from build123d import *

# Parameters (mm, degrees)
F1_DEPTH  = 45
F3_D      = 5
F3_DEPTH  = 20
F3_TIP    = 1.5021515476
F5_D      = 5
F5_DEPTH  = 20
F5_TIP    = 1.5021515476
F8_D      = 5
F8_DEPTH  = 20
F8_TIP    = 1.5021515476
F10_D     = 5
F10_DEPTH = 20
F10_TIP   = 1.5021515476


with BuildPart() as f1:
    # F0 (on Front) → F1 (new body)
    with BuildSketch(Plane.XZ):
        Polygon((50, 20), (20, 20), (10, 20), (0, 10), (-10, 20), (-20, 20), (-50, 20), (-50, 0), (-50, -10), (50, -10), (50, 0), align=None)
    extrude(amount=F1_DEPTH)

    # F3
    with Locations(Plane.XY.offset(20)):
        with Locations((35, -35)):
            Hole(F3_D / 2, depth=F3_DEPTH)
            with Locations((0, 0, -(F3_DEPTH + F3_TIP / 2))):  # 118° drill point
                Cone(0, F3_D / 2, F3_TIP, mode=Mode.SUBTRACT)

    # F5
    with Locations(Plane.XY.offset(20)):
        with Locations((35, -10)):
            Hole(F5_D / 2, depth=F5_DEPTH)
            with Locations((0, 0, -(F5_DEPTH + F5_TIP / 2))):  # 118° drill point
                Cone(0, F5_D / 2, F5_TIP, mode=Mode.SUBTRACT)

    # F8
    with Locations(Plane.XY.offset(20)):
        with Locations((-35, -35)):
            Hole(F8_D / 2, depth=F8_DEPTH)
            with Locations((0, 0, -(F8_DEPTH + F8_TIP / 2))):  # 118° drill point
                Cone(0, F8_D / 2, F8_TIP, mode=Mode.SUBTRACT)

    # F10
    with Locations(Plane.XY.offset(20)):
        with Locations((-34.9459722638, -9.987832047)):
            Hole(F10_D / 2, depth=F10_DEPTH)
            with Locations((0, 0, -(F10_DEPTH + F10_TIP / 2))):  # 118° drill point
                Cone(0, F10_D / 2, F10_TIP, mode=Mode.SUBTRACT)


solid = f1.part
Can you work these out from the model? Positions are in its coordinate system, mm. A direction names the side the tool comes from. Coordinates: 2 decimals unless noted, no trailing zeros. Write each loop counter-clockwise with the first axis right and the second up, starting at its lowest first coordinate (ties: lowest second). Pieces come first, ordered by that corner, then holes. Notation, with made-up numbers: M -8.75,9 L 3.25,9 A22 ccw 3.25,36 Z; hole C 51,65 d2. An arc over 180 degrees is marked long. Use one line per item in the form item = value.
Q1. For faces 1 (the flat face through (5, -22, 15)), 2 (the cylindrical face through (32.69, -10.96, 9.86)), 3 (the flat face through (-50, -22, 5)), which set-ups out of +Z, -Z, +X, -X, +Y, -Y let a thin tool reach every point of the face, with its end or its side?
Model answer:
face_1 = +Z, +Y, -Y
face_2 = +Z
face_3 = +Z, -Z, -X, +Y, -Y
Q2. For P1, Ø4, axis at x = -34.95, y = -9.99, coming from the +Z side, with a flat end and sliding along its axis, tell me the tip position at first contact or that it passes through.
Model answer:
P1 = -0.3
Q3. I need wall thicknesses on line 1 along Y through (x, z) = (-35, 12.5); line 2 along X through (y, z) = (-35, 9.25); line 3 along X through (y, z) = (-10, 4.5). Which ranges of each line are inside material? Lowest first, please. Write a range as from..to.
Model answer:
line_1 = -45..-37.5, -32.5..-12.49, -7.49..0
line_2 = -50..-37.5, -32.5..32.5, 37.5..50
line_3 = -50..-37.45, -32.45..32.5, 37.5..50
Q4. If we section it at A-A (y = -6): Write out the boundary of the cut face in (x, z), then the cut area to 3 significant figures.
Model answer:
outline = M -50,-10 L 50,-10 L 50,20 L 10,20 L 0,10 L -10,20 L -50,20 Z
area = 2,900 mm^2
Q5. If we section it at B-B (z = 11.75): Write out the boundary of the cut face in (x, y), then the cut area to 3 significant figures.
Model answer:
outline = M -50,-45 L -1.75,-45 L -1.75,0 L -50,0 Z; M 1.75,-45 L 50,-45 L 50,0 L 1.75,0 Z; hole C -35,-35 d5; hole C -34.95,-9.99 d5; hole C 35,-35 d5; hole C 35,-10 d5
area = 4,260 mm^2
Q6. We'd pull the mould along Y, two halves only. Please class faces 4 (the flat face through (50, -22, 5)), 5 (the cylindrical face through (32.615, -34.249, 9.86)), 6 (the flat face through (-1, -45, 5)): +Y half, -Y half, draft (parallel to the pull), parting line (faces both ways), or undercut.
Model answer:
face_4 = draft
face_5 = undercut
face_6 = -Y half
Q7. If we section it at D-D (z = 2.25): Write out the boundary of the cut face in (x, y), then the cut area to 3 significant figures.
Model answer:
outline = M -50,-45 L 50,-45 L 50,0 L -50,0 Z; hole C -35,-35 d5; hole C -34.95,-9.99 d5; hole C 35,-35 d5; hole C 35,-10 d5
area = 4,420 mm^2
Q8. If we section it at C-C (x = -5): Write out the boundary of the cut face in (y, z).
Model answer:
outline = M -45,-10 L 0,-10 L 0,15 L -45,15 Z
